from build123d import *

# Parameters (mm, degrees)
SKETCH_1_R               = 48.25
EXTRUDE_2_DEPTH          = 42.4
SKETCH_2_R               = 1.75
CUT_EXTRUDE_1_DEPTH      = 81.336075334
PATTERN_CIRCULAR_2_COUNT = 8
SKETCH_4_R               = 19
EXTRUDE_4_DEPTH          = 50
SKETCH_5_R               = 2
CUT_EXTRUDE_2_DEPTH      = 119.852103634
PATTERN_CIRCULAR_3_COUNT = 6


with BuildPart() as part:
    # 草图1 → 凸台-拉伸2 (new body)
    with BuildSketch(Plane(origin=(0, 0, 0), x_dir=(1, 0, 0), z_dir=(0, 1, 0))):
        with Locations(Location((0, 0, 0), (0, 0, 270))):
            Circle(SKETCH_1_R)
    extrude(amount=EXTRUDE_2_DEPTH)

    # 草图2 → 切除-拉伸1 (cut, symmetric)
    with BuildSketch(Plane(origin=(0, 42.4, 0), x_dir=(1, 0, 0), z_dir=(0, 1, 0))):
        with Locations(Location((20.051879178, 37.472284978, 0), (0, 0, 270))):
            Circle(SKETCH_2_R)
    cut_extrude_1 = extrude(amount=CUT_EXTRUDE_1_DEPTH, both=True, mode=Mode.SUBTRACT)

    # 阵列(圆周)2: 切除-拉伸1 ×8 about axis
    pattern_circular_2_axis = Axis((0, 0, 0), (0, 1, 0))
    for i in range(1, PATTERN_CIRCULAR_2_COUNT):
        add(cut_extrude_1.rotate(pattern_circular_2_axis, i * 360 / PATTERN_CIRCULAR_2_COUNT), mode=Mode.SUBTRACT)

    # 草图4 → 凸台-拉伸4 (add, symmetric)
    with BuildSketch(Plane.XY):
        with Locations(Location((0, 21.2, 0), (0, 0, 180))):
            Circle(SKETCH_4_R)
    extrude(amount=EXTRUDE_4_DEPTH, both=True)

    # 草图5 → 切除-拉伸2 (cut, symmetric)
    with BuildSketch(Plane.XY.offset(50)):
        with Locations((0, 37.2)):
            Circle(SKETCH_5_R)
    cut_extrude_2 = extrude(amount=CUT_EXTRUDE_2_DEPTH, both=True, mode=Mode.SUBTRACT)

    # 阵列(圆周)3: 切除-拉伸2 ×6 about axis
    pattern_circular_3_axis = Axis((0, 21.2, 0), (0, 0, 1))
    for i in range(1, PATTERN_CIRCULAR_3_COUNT):
        add(cut_extrude_2.rotate(pattern_circular_3_axis, i * 360 / PATTERN_CIRCULAR_3_COUNT), mode=Mode.SUBTRACT)


solid = part.part
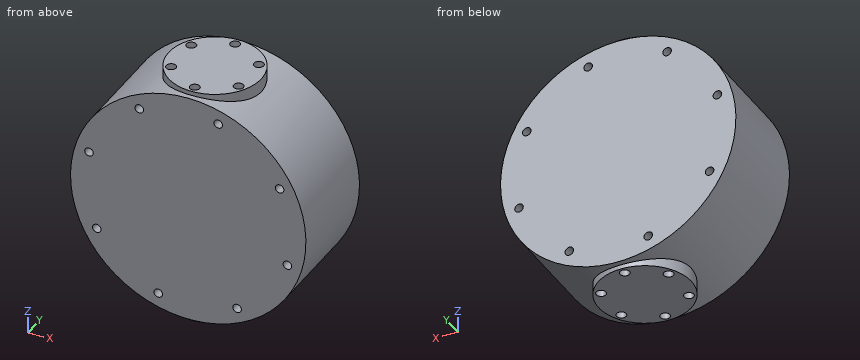
Input: part model. Units: mm. Frame: model coordinates. Give positions to 0.01 mm unless a question says otherwise; leave off trailing zeros. Order: outer loops, then holes, each group sorted by start corner. A loop starts at its lowest first (then second) coordinate and runs counter-clockwise, first axis right, second up. Notation, with made-up numbers: M -30,-27 L -21,-27 A22 cw -21,1 Z; hole C 55,0.5 d7. An arc over 180 degrees is marked long. Answer as a JSON object with one key per item and string values.
1. Cut plane C-C, the plane z = 6.5. Output: boundary loops of the cut face in (x, y), and give its area (3 significant figures).
Result sheet:
{"outline": "M -47.81,0 L 47.81,0 L 47.81,42.4 L -47.81,42.4 Z; hole C -13.86,13.2 d4; hole C -13.86,29.2 d4; hole C 0,5.2 d4; hole C 0,37.2 d4; hole C 13.86,13.2 d4; hole C 13.86,29.2 d4", "area": "3,980 mm²"}
2. First-contact query: P1, Ø1, axis at x = -37.5, y = 7, coming from the -Z side; P2, Ø4, axis at x = -40.68, z = 12.32, coming from the +Y side; P3, Ø3, axis at x = 12.32, z = 40.68, coming from the +Y side; P4, Ø3, axis at y = 9, z = -20, coming from the +X side. Flat tips, straight axial feed; report the tip coordinate or a pass-through.
Result sheet:
{"P1": "z = -30.97", "P2": "y = 42.4", "P3": "y = 36.82", "P4": "x = 44.56"}
3. Cut plane B-B, the plane y = 29.2. State how many separate pieces and enclosed holes the cut face has, and give its area (3 significant figures).
Result sheet:
{"separate pieces": "3", "enclosed holes": "6", "area": "6,650 mm²"}
4. Cut plane D-D, the plane y = 23. Output: boundary loops of the cut face in (x, z).
Result sheet:
{"outline": "M -18.91,-50 L 18.91,-50 L 18.91,-44.39 A48.25 ccw 18.91,44.39 L 18.91,50 L -18.91,50 L -18.91,44.39 A48.25 ccw -18.91,-44.39 Z; hole C -40.68,12.32 d3.5; hole C -37.47,-20.05 d3.5; hole M -18.91,36.14 L -18.91,38.8 A1.75 ccw long Z; hole M 18.91,-38.8 A1.75 ccw long 18.91,-36.14 Z; hole C 37.47,20.05 d3.5; hole C 40.68,-12.32 d3.5"}
5. Ray query, line 1 (Y direction, x = 0, z = 25); line 2 (Z direction, x = -23, y = 24); line 3 (X direction, y = 7, z = -16). Return the intervals inside material, ascending. Write a range as [from, to].
Result sheet:
{"line 1": "[0, 3.2], [7.2, 35.2], [39.2, 42.4]", "line 2": "[-42.42, 42.42]", "line 3": "[-45.52, -0.87], [0.87, 45.52]"}
6. Cut plane A-A, the plane x = 0. Output: boundary loops of the cut face in (y, z), and give its area (3 significant figures).
Result sheet:
{"outline": "M 0,-48.25 L 2.2,-48.25 L 2.2,-50 L 3.2,-50 L 3.2,50 L 2.2,50 L 2.2,48.25 L 0,48.25 Z; M 7.2,-50 L 35.2,-50 L 35.2,50 L 7.2,50 Z; M 39.2,-50 L 40.2,-50 L 40.2,-48.25 L 42.4,-48.25 L 42.4,48.25 L 40.2,48.25 L 40.2,50 L 39.2,50 Z", "area": "3,420 mm²"}
